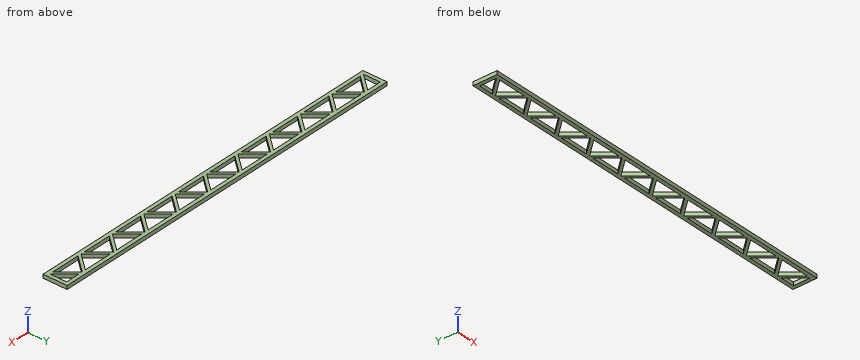
```python
from build123d import *

# Parameters (mm, degrees)
F1_DEPTH = 1.27


with BuildPart() as f1:
    # F0 (on Top) → F1 (new body)
    with BuildSketch(Plane.XY):
        Polygon((19.046307, 4.947169), (-111.282837, 4.947169), (-111.282837, -3.485631), (19.046307, -3.485631), (19.046307, -2.215631), align=None)
        Polygon((-110.012837, -2.215631), (-110.012837, 3.677169), (-104.890304, 3.677169), align=None, mode=Mode.SUBTRACT)
        Polygon((-98.503923, -2.215631), (-108.742837, -2.215631), (-103.62338, 3.677169), align=None, mode=Mode.SUBTRACT)
        Polygon((-92.11139, 3.677169), (-97.233923, -2.215631), (-102.356456, 3.677169), align=None, mode=Mode.SUBTRACT)
        Polygon((-85.725008, -2.215631), (-95.963923, -2.215631), (-90.844466, 3.677169), align=None, mode=Mode.SUBTRACT)
        Polygon((-79.332476, 3.677169), (-84.455008, -2.215631), (-89.577541, 3.677169), align=None, mode=Mode.SUBTRACT)
        Polygon((-72.946094, -2.215631), (-83.185008, -2.215631), (-78.065551, 3.677169), align=None, mode=Mode.SUBTRACT)
        Polygon((-66.553561, 3.677169), (-71.676094, -2.215631), (-76.798627, 3.677169), align=None, mode=Mode.SUBTRACT)
        Polygon((-70.406094, -2.215631), (-65.286637, 3.677169), (-60.16718, -2.215631), align=None, mode=Mode.SUBTRACT)
        Polygon((-53.774647, 3.677169), (-58.89718, -2.215631), (-64.019712, 3.677169), align=None, mode=Mode.SUBTRACT)
        Polygon((-47.388265, -2.215631), (-57.62718, -2.215631), (-52.507722, 3.677169), align=None, mode=Mode.SUBTRACT)
        Polygon((-40.995732, 3.677169), (-46.118265, -2.215631), (-51.240798, 3.677169), align=None, mode=Mode.SUBTRACT)
        Polygon((-44.848265, -2.215631), (-39.728808, 3.677169), (-34.609351, -2.215631), align=None, mode=Mode.SUBTRACT)
        Polygon((-28.216818, 3.677169), (-33.339351, -2.215631), (-38.461884, 3.677169), align=None, mode=Mode.SUBTRACT)
        Polygon((-32.069351, -2.215631), (-26.949893, 3.677169), (-21.830436, -2.215631), align=None, mode=Mode.SUBTRACT)
        Polygon((-15.437903, 3.677169), (-20.560436, -2.215631), (-25.682969, 3.677169), align=None, mode=Mode.SUBTRACT)
        Polygon((-19.290436, -2.215631), (-14.170979, 3.677169), (-9.051522, -2.215631), align=None, mode=Mode.SUBTRACT)
        Polygon((-2.658989, 3.677169), (-7.781522, -2.215631), (-12.904055, 3.677169), align=None, mode=Mode.SUBTRACT)
        Polygon((3.727393, -2.215631), (-6.511522, -2.215631), (-1.392065, 3.677169), align=None, mode=Mode.SUBTRACT)
        Polygon((10.119926, 3.677169), (4.997393, -2.215631), (-0.12514, 3.677169), align=None, mode=Mode.SUBTRACT)
        Polygon((6.267393, -2.215631), (11.38685, 3.677169), (16.506307, -2.215631), align=None, mode=Mode.SUBTRACT)
        Polygon((17.776307, 3.677169), (17.776307, -2.215631), (12.653774, 3.677169), align=None, mode=Mode.SUBTRACT)
    extrude(amount=F1_DEPTH)


solid = f1.part
```
Geometry check sheet. Reference: the model listing, model coordinates, mm. Give positions to 0.01 mm unless a question says otherwise; leave off trailing zeros. Write each loop counter-clockwise with the first axis right and the second up, starting at its lowest first coordinate (ties: lowest second). Pieces come first, ordered by that corner, then holes. Notation, with made-up numbers: (7, -39.75) - (65, -39.75) arc R19 cw to (65, -34.75) - close; hole circle Ø11 at (15, 23). An arc over 180 degrees is marked (long way). Use a Markdown table: item, result.
Q1. Section check A-A, the plane x = -50. Enter the section's corners in (y, z), then the cut area to 3 significant figures.
Computed:
| item | result |
|---|---|
| outline | (-3.49, 0) - (-2.22, 0) - (-2.22, 1.27) - (-3.49, 1.27) - close; (0.79, 0) - (2.25, 0) - (2.25, 1.27) - (0.79, 1.27) - close; (3.68, 0) - (4.95, 0) - (4.95, 1.27) - (3.68, 1.27) - close |
| area | 5.08 mm² |
Q2. Section check B-B, the plane z = 0.35. Give the number of separate pieces and of enclosed holes in the cut face, then the cut area to 4 significant figures.
Computed:
| item | result |
|---|---|
| separate pieces | 1 |
| enclosed holes | 21 |
| area | 495.5 mm² |
Q3. Thickness scan on L1, parallel to Y at x = -69, z = 0.3; L2, parallel to Y at x = -50.5, z = 0.4; L3, parallel to Y at x = 11.5, z = 0.9. Record the ranges inside material, lowest first. Write a range as [from, to].
Computed:
| item | result |
|---|---|
| L1 | y = [-3.49, -2.22], [-0.6, 0.86], [3.68, 4.95] |
| L2 | y = [-3.49, -2.22], [1.37, 2.82], [3.68, 4.95] |
| L3 | y = [-3.49, -2.22], [3.55, 4.95] |
